Here's how the part is built. I have some questions about the finished solid (model axes, mm). Face numbers are marked on the shaded views. A direction names the side the tool comes from. Round coordinates to 2 decimals unless told otherwise and drop trailing zeros. Write each loop counter-clockwise with the first axis right and the second up, starting at its lowest first coordinate (ties: lowest second). Pieces come first, ordered by that corner, then holes. Notation, with made-up numbers: M 52,14 L 82,14 A20 ccw 82,21 Z; hole C -1,-25.5 d7. An arc over 180 degrees is marked long. Use one line per item in the form item = value. Start each with the question number.
Q1. I need wall thicknesses on line 1 along X through (y, z) = (-48, 17); line 2 along X through (y, z) = (-37.5, 38); line 3 along Z through (x, y) = (52, -67). Which ranges of each line are inside material? Lowest first, please. Write a range as from..to.
Q2. I want a section at D-D on y = -47.5. List the corners of the cut face in (x, z) for me (1 decimal), and give its area (3 significant figures).
Q3. I want a section at B-B on x = 73. List the corners of the cut face in (y, z) for me.
Q4. For the marked faces 4, 5, 6, 7 and 8, which set-ups out of +Z, -Z, +X, -X, +Y, -Y let a thin tool reach every point of the face, with its end or its side?
Q5. I want a section at A-A on y = -30. State how many separate pieces and enclosed holes the cut face has, and give its area (3 significant figures).
Q6. We'd pull the mould along X, two halves only. Please class the marked faces 1, 2 and 3: +X half, -X half, draft (parallel to the pull), parting line (faces both ways), or undercut.
Q7. I'm going to push flat-ended pins straight in: pin 1 Ø6.5 at (x, z) = (7.25, 23.5) entering from -Y; pin 2 Ø24.5 at (x, z) = (34.5, 28.5) entering from -Y; pin 3 Ø6 at (y, z) = (-21.5, 19.5) entering from +X; pin 4 Ø5.5 at (y, z) = (-32, 43.5) entering from -X. Where does each tip first touch, or does it pass through?
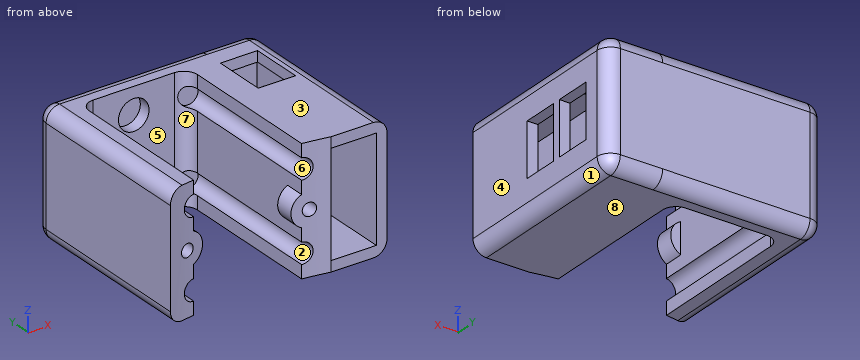
```python
from build123d import *

# Parameters (mm, degrees)
SKETCH1_W           = 60.452
SKETCH1_H           = 71.12
BOSS_EXTRUDE1_DEPTH = 46.99
SKETCH2_W           = 40.64
SKETCH2_H           = 85.320739167
CUT_EXTRUDE1_DEPTH  = 46.99
SKETCH3_R           = 2.44475
CUT_EXTRUDE2_DEPTH  = 30.734
SKETCH5_R           = 6.35
BOSS_EXTRUDE4_DEPTH = 9.652
SKETCH3_5_R         = 2.44475
CUT_EXTRUDE3_DEPTH  = 38.1
FILLET1_R           = 5.08
SKETCH9_R           = 5.737107227
CUT_EXTRUDE6_DEPTH  = 4.572
SKETCH10_R          = 3.900639461
CUT_EXTRUDE10_DEPTH = 62.23
SKETCH8_R           = 152.4
CUT_EXTRUDE11_DEPTH = 55.372
SKETCH11_W          = 46.99
SKETCH11_H          = 65.461586673
BOSS_EXTRUDE6_DEPTH = 21
SKETCH12_W          = 17
SKETCH12_H          = 38.99
CUT_EXTRUDE12_DEPTH = 63
FILLET2_R           = 5.08
SKETCH25_W          = 20
SKETCH25_H          = 14
CUT_EXTRUDE13_DEPTH = 10
SKETCH26_W          = 14
SKETCH26_H          = 20
CUT_EXTRUDE14_DEPTH = 10


with BuildPart() as part:
    # Sketch1 → Boss-Extrude1 (new body)
    with BuildSketch(Plane.XY):
        with Locations((30.226, -35.56)):
            Rectangle(SKETCH1_W, SKETCH1_H)
    extrude(amount=BOSS_EXTRUDE1_DEPTH)

    # Sketch2 → Cut-Extrude1 (cut)
    with BuildSketch(Plane.XY.offset(46.99)):
        with Locations((30.226, -51.550369584)):
            Rectangle(SKETCH2_W, SKETCH2_H)
    extrude(amount=-CUT_EXTRUDE1_DEPTH, mode=Mode.SUBTRACT)

    # Sketch3 → Cut-Extrude2 (cut)
    with BuildSketch(Plane.XZ.offset(71.12)):
        with Locations((53.2003, 23.495)):
            Circle(SKETCH3_R)
        with Locations((7.2517, 23.495)):
            Circle(SKETCH3_R)
    extrude(amount=-CUT_EXTRUDE2_DEPTH, mode=Mode.SUBTRACT)

    # Sketch5 → Boss-Extrude4 (add)
    with BuildSketch(Plane.XZ.offset(71.12)):
        with Locations((7.2517, 23.495)):
            Circle(SKETCH5_R)
        with Locations((53.2003, 23.495)):
            Circle(SKETCH5_R)
    extrude(amount=-BOSS_EXTRUDE4_DEPTH)

    # Sketch3<5> → Cut-Extrude3 (cut)
    with BuildSketch(Plane.XZ.offset(71.12)):
        with Locations((53.2003, 23.495)):
            Circle(SKETCH3_5_R)
        with Locations((7.2517, 23.495)):
            Circle(SKETCH3_5_R)
    extrude(amount=-CUT_EXTRUDE3_DEPTH, mode=Mode.SUBTRACT)

    # Fillet1
    fillet1_edges = [part.edges().sort_by_distance(p)[0] for p in [
        (30.226, 0, 46.99),
        (50.546, -8.89, 23.495),
        (9.906, -8.89, 23.495),
        (0, -35.56, 46.99),
        (30.226, 0, 0),
        (0, -35.56, 0),
        (0, 0, 23.495),
    ]]
    fillet(fillet1_edges, radius=FILLET1_R)

    # Sketch9 → Cut-Extrude6 (cut)
    with BuildSketch(Plane.XZ.offset(8.89)):
        with Locations((30.226, 37.042280921)):
            Circle(SKETCH9_R)
        with Locations((30.226, 9.947719079)):
            Circle(SKETCH9_R)
    extrude(amount=-CUT_EXTRUDE6_DEPTH, mode=Mode.SUBTRACT)

    # Sketch10 → Cut-Extrude10 (cut)
    with BuildSketch(Plane(origin=(0, -71.12, 0), x_dir=(-1, 0, 0), z_dir=(0, -1, 0))):
        with Locations((-9.906, -38.126819309)):
            Circle(SKETCH10_R)
        with Locations((-9.906, -8.863180691)):
            Circle(SKETCH10_R)
        with Locations((-50.546, -38.126819309)):
            Circle(SKETCH10_R)
        with Locations((-50.546, -8.863180691)):
            Circle(SKETCH10_R)
    extrude(amount=-CUT_EXTRUDE10_DEPTH, mode=Mode.SUBTRACT)

    # Sketch8 → Cut-Extrude11 (cut)
    with BuildSketch(Plane.XY.offset(46.99)):
        with Locations((30.473524119, -219.963977846)):
            Circle(SKETCH8_R)
    extrude(amount=-CUT_EXTRUDE11_DEPTH, mode=Mode.SUBTRACT)

    # Sketch11 → Boss-Extrude6 (add)
    with BuildSketch(Plane(origin=(60.452, 0, 0), x_dir=(0, 0, -1), z_dir=(1, 0, 0))):
        with BuildLine():
            Line((-46.99, -5.08), (0, -5.08))
            ThreePointArc((0, -5.08), (-1.487897552, -1.487897552), (-5.08, 0))
            Line((-5.08, 0), (-41.91, 0))
            ThreePointArc((-41.91, 0), (-45.502102448, -1.487897552), (-46.99, -5.08))
        make_face()
        with Locations((-23.495, -37.810793336)):
            Rectangle(SKETCH11_W, SKETCH11_H)
    extrude(amount=BOSS_EXTRUDE6_DEPTH)

    # Sketch12 → Cut-Extrude12 (cut)
    with BuildSketch(Plane(origin=(0, -70.541586673, 0), x_dir=(-1, 0, 0), z_dir=(0, -1, 0))):
        with Locations((-68.952, -23.495)):
            Rectangle(SKETCH12_W, SKETCH12_H)
    extrude(amount=-CUT_EXTRUDE12_DEPTH, mode=Mode.SUBTRACT)

    # Fillet2
    fillet2_edges = [part.edges().sort_by_distance(p)[0] for p in [
        (81.452, -1.487897552, 45.502102448),
        (81.452, -37.810793337, 46.99),
        (81.452, -37.810793337, 0),
        (81.452, -1.487897552, 1.487897552),
        (81.452, 0, 23.495),
    ]]
    fillet(fillet2_edges, radius=FILLET2_R)

    # Sketch25 → Cut-Extrude13 (cut)
    with BuildSketch(Plane(origin=(81.452, 0, 0), x_dir=(0, 0, -1), z_dir=(1, 0, 0))):
        with Locations((-23.49, -18)):
            Rectangle(SKETCH25_W, SKETCH25_H)
        with Locations((-23.49, -35)):
            Rectangle(SKETCH25_W, SKETCH25_H)
    extrude(amount=-CUT_EXTRUDE13_DEPTH, mode=Mode.SUBTRACT)

    # Sketch26 → Cut-Extrude14 (cut)
    with BuildSketch(Plane.XY.offset(46.99)):
        with Locations((67.546, -22)):
            Rectangle(SKETCH26_W, SKETCH26_H)
    extrude(amount=-CUT_EXTRUDE14_DEPTH, mode=Mode.SUBTRACT)


solid = part.part
```
Reported:
q1.line_1 = 0..9.91, 50.55..60.45, 77.45..81.45
q1.line_2 = 0..6.01, 54.44..60.45, 77.45..81.45
q1.line_3 = 0..5.24, 12.48..21.37, 25.62..34.51, 41.75..46.99
q2.outline = M 0,5.1 A5.1 ccw 5.1,0 L 9.9,0 L 9.9,5 A3.9 cw 9.9,12.8 L 9.9,34.2 A3.9 cw 9.9,42 L 9.9,47 L 5.1,47 A5.1 ccw 0,41.9 Z; M 50.5,0 L 76.4,0 A5.1 ccw 81.5,5.1 L 81.5,41.9 A5.1 ccw 76.4,47 L 50.5,47 L 50.5,42 A3.9 cw 50.5,34.2 L 50.5,12.8 A3.9 cw 50.5,5 Z; hole C 7.3,23.5 d4.9; hole C 53.2,23.5 d4.9; hole M 60.5,4 L 77.5,4 L 77.5,43 L 60.5,43 Z
q2.area = 1,100 mm^2
q3.outline = M -70.54,0 L -5.08,0 A5.08 ccw 0,5.08 L 0,41.91 A5.08 ccw -5.08,46.99 L -12,46.99 L -12,42.99 L -7.54,42.99 L -7.54,4 L -70.54,4 Z; M -70.54,42.99 L -32,42.99 L -32,46.99 L -70.54,46.99 Z
q4.face_4 = +Z, -Z, +X, +Y, -Y
q4.face_5 = +Z, -Z, -Y
q4.face_6 = -Y
q4.face_7 = +Z, -Z
q4.face_8 = -Z, +X, -X, +Y, -Y
q5.separate_pieces = 3
q5.enclosed_holes = 0
q5.area = 1,000 mm^2
q6.face_1 = +X half
q6.face_2 = undercut
q6.face_3 = draft
q7.pin_1 = -69.88
q7.pin_2 = -9.05
q7.pin_3 = 60.45
q7.pin_4 = 0
